from build123d import *

# Parameters (mm, degrees)
SKETCH1_R           = 12.7
SKETCH1_R_2         = 2.25
BOSS_EXTRUDE1_DEPTH = 3.175


with BuildPart() as part:
    # Sketch1 → Boss-Extrude1 (new body)
    with BuildSketch(Plane(origin=(0, 0, 0), x_dir=(1, 0, 0), z_dir=(0, 1, 0))):
        with BuildLine():
            ThreePointArc((-41.632787539, 12.230172128), (-47.862074133, -1.911659432), (-38.249546762, -14.011028378))
            ThreePointArc((-38.249546762, -14.011028378), (-23.068421331, -24.399712606), (-14.524270984, -40.690471465))
            ThreePointArc((-14.524270984, -40.690471465), (0, -52.098148446), (14.524270984, -40.690471465))
            ThreePointArc((14.524270984, -40.690471465), (23.068421331, -24.399712606), (38.249546762, -14.011028378))
            ThreePointArc((38.249546762, -14.011028378), (47.862074133, -1.911659432), (41.632787539, 12.230172128))
            ThreePointArc((41.632787539, 12.230172128), (0, 25.4), (-41.632787539, 12.230172128))
        make_face()
        Circle(SKETCH1_R, mode=Mode.SUBTRACT)
        with Locations((-33.0348, 0)):
            Circle(SKETCH1_R_2, mode=Mode.SUBTRACT)
        with Locations((33.0348, 0)):
            Circle(SKETCH1_R_2, mode=Mode.SUBTRACT)
        with Locations((0, -37.148148446)):
            Circle(SKETCH1_R_2, mode=Mode.SUBTRACT)
    extrude(amount=BOSS_EXTRUDE1_DEPTH)


solid = part.part
For this review, take the finished solid that the model builds, in its own axes (mm). Round coordinates to 2 decimals unless told otherwise and drop trailing zeros. Order: outer loops, then holes, each group sorted by start corner. A loop starts at its lowest first (then second) coordinate and runs counter-clockwise, first axis right, second up. Notation, with made-up numbers: M 11,56 L 60,56 A10 cw 60,75 Z; hole C 8.25,61 d11. An arc over 180 degrees is marked long. Write each question's results on one line, items separated by ' | '. Start each with the question number.
1. Add section A-A (z = 0). State the section outline as (x, y) points (3 decimals).
2. Add section D-D (z = 10.5). State the section outline as (x, y) points (3 decimals).
3. Add section C-C (y = 2.25). State the section outline as (x, z) points.
4. Draft analysis for pull direction Z (two halves, no side actions). For faces 1 (the face through (-1, 0, 13)), 2 (the face through (-23.24, 1.57, 24.21)), 3 (the face through (-0.293, 1.565, 34.917)), 4 (the face through (30.787, 1.565, -0.099)), state which applies: pulls with the +Z half, pulls with the -Z half, needs draft (parallel to the pull), parting line crosses it, or undercut.
5. Add section B-B (x = 0). State the section outline as (y, z) points (3 decimals), then the cut area to 3 significant figures.
6. To check wall thickness, follow L1, parallel to X at y = 2.35, z = 0; L2, parallel to Z at x = 0, y = 2.1; L3, parallel to Z at x = -1.5, y = 2.2. State the ranges of each line that lie inside material, in increasing order. Write a range as [from, to].
7. Clearance check with a flat-ended pin moving along its axis: pin 1 Ø1.5 at (y, z) = (1, 41.5) entering from +X. State where the tip first meets the part, or that it passes through.
Output values:
1) outline: M -47.985,0 L -35.285,0 L -35.285,3.175 L -47.985,3.175 Z; M -30.785,0 L -12.7,0 L -12.7,3.175 L -30.785,3.175 Z; M 12.7,0 L 30.785,0 L 30.785,3.175 L 12.7,3.175 Z; M 35.285,0 L 47.985,0 L 47.985,3.175 L 35.285,3.175 Z
2) outline: M -43.677,0 L -7.144,0 L -7.144,3.175 L -43.677,3.175 Z; M 7.144,0 L 43.677,0 L 43.677,3.175 L 7.144,3.175 Z
3) outline: M -41.63,-12.23 A72.39 ccw 41.63,-12.23 A14.95 ccw 38.25,14.01 A38.1 cw 14.52,40.69 A14.95 ccw -14.52,40.69 A38.1 cw -38.25,14.01 A14.95 ccw Z; hole C -33.03,0 d4.5; hole C 0,0 d25.4; hole C 0,37.15 d4.5; hole C 33.03,0 d4.5
4) face 1: needs draft | face 2: pulls with the +Z half | face 3: undercut | face 4: undercut
5) outline: M 0,-25.4 L 3.175,-25.4 L 3.175,-12.7 L 0,-12.7 Z; M 0,12.7 L 3.175,12.7 L 3.175,34.898 L 0,34.898 Z; M 0,39.398 L 3.175,39.398 L 3.175,52.098 L 0,52.098 Z | area: 151 mm^2
6) L1: [-47.98, -35.28], [-30.78, -12.7], [12.7, 30.78], [35.28, 47.98] | L2: [-25.4, -12.7], [12.7, 34.9], [39.4, 52.1] | L3: [-25.38, -12.61], [12.61, 35.47], [38.83, 52.02]
7) pin 1: x = 14.51
